Geometry: see drawing. Coordinates: mm, zero at the bounding-box minimum. Give positions to 0.01 mm unless a question says otherwise; leave off trailing zeros. Loops run counter-clockwise (first coordinate to the right, second up) from the corner with the lowest first, then second, coordinate; pieces in that order, holes last. Notation, with made-up numbers: M 40.25,54.25 L 71.25,54.25 A22 cw 71.25,91.25 Z; hole C -8,-20 d8. An arc over 180 degrees is marked long. Use CSV: the item, a comma, the result in double quotes. Start each with the question number.
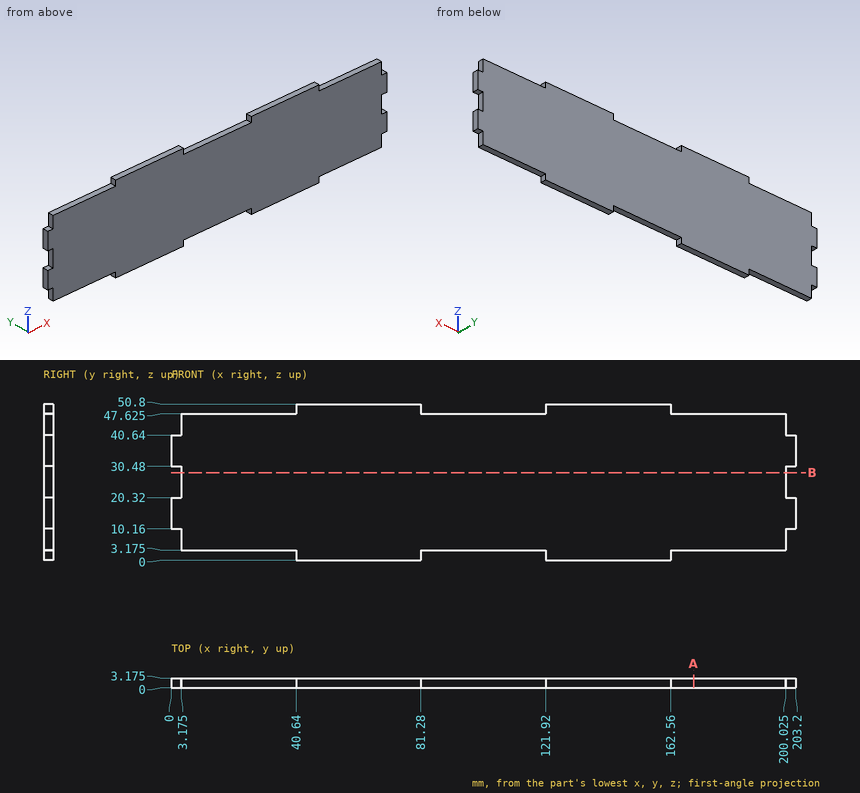
Item 1: Section A-A (x = 170). Output: boundary loops of the cut face in (y, z) (3 decimals).
Item 2: Section B-B (z = 28.5). Output: boundary loops of the cut face in (x, y) (3 decimals), then the cut area to 3 significant figures.
Item 3: First-contact query: pin 1 Ø1 at (y, z) = (2.5, 8.5) entering from -X (3 decimals); pin 2 Ø1 at (y, z) = (2, 1.5) entering from +X; pin 3 Ø1 at (y, z) = (0.5, 12.5) entering from -X; pin 4 Ø1.6 at (x, y) = (202, 1.5) entering from -Z. Flat tips, straight axial feed; report the tip coordinate or a pass-through.
Item 4: Material intervals for line 1 (X direction, y = 2.15, z = 45) (3 decimals); line 2 (Z direction, x = 33, y = 1.2) (3 decimals), sorted ascending.
Recorded:
1,outline,"M 0,3.175 L 3.175,3.175 L 3.175,47.625 L 0,47.625 Z"
2,outline,"M 3.175,0 L 200.025,0 L 200.025,3.175 L 3.175,3.175 Z"
2,area,"625 mm²"
3,pin 1,"x = 3.175"
3,pin 2,"x = 162.56"
3,pin 3,"x = 0"
3,pin 4,"z = 10.16"
4,line 1,"3.175 to 200.025"
4,line 2,"3.175 to 47.625"
